Design review of the part built by this model. Coordinates are the model's own, in mm. A direction names the side the tool comes from. Coordinates: 2 decimals unless noted, no trailing zeros. Write each loop counter-clockwise with the first axis right and the second up, starting at its lowest first coordinate (ties: lowest second). Pieces come first, ordered by that corner, then holes.
Q1. Add section B-B, the plane y = 41. Give the boundary of the cut face in (x, z).
Q2. Clearance check with flat-ended pins moving along their axes: pin 1 Ø3 at (y, z) = (10, -4) entering from +X; pin 2 Ø1.8 at (y, z) = (60, -2.5) entering from -X; pin 3 Ø2.5 at (x, z) = (295.5, -3) entering from -Y. State where each tip first meets the part, or that it passes through.
Q3. Add section D-D, the plane z = -1.5. Give the number of separate pieces and of enclosed holes in the cut face, plus the area to 3 significant figures.
Q4. Machinability: for faces 5 (the face through (170, -3, -3)), 6 (the face through (3, 45, -3)), 7 (the face through (294, 57, -3)), 8 (the face through (3, 25, -3)), which of the approach directions +Z, -Z, +X, -X, +Y, -Y give a long, thin tool a straight path to every point of the face, cutting with its end or side? Answer none if there is none.
Q5. Add section A-A, the plane x = 179. Give the boundary of the cut face in (y, z), plus the area to 3 significant figures.
Q6. Add section C-C, the plane x = 80. Give the boundary of the cut face in (y, z), plus the area to 3 significant figures.
Q7. The part is to be moulded in two halves that separate along Y. For faces 1 (the face through (241.102, 46.827, -2.958)), 2 (the face through (68, 0, -3)), 3 (the face through (130, -3, -3)), 4 (the face through (148, 70, -3)), say which applies: +Y half, -Y half, draft (parallel to the pull), parting line (faces both ways), or undercut.
Q8. To check wall thickness, follow probe 1 along Y at (x, z) = (106, -3.85); probe 2 along Y at (x, z) = (131, -4.15); probe 3 along X at (y, z) = (37, -3.7). State the ranges of each line that lie inside material, in increasing order.
from build123d import *

# Parameters (mm, degrees)
SKETCH1_W           = 300
SKETCH1_H           = 70
FRONT_DEPTH         = 6
SKETCH2_W           = 6
SKETCH2_H           = 25
SKETCH2_R           = 4
MOUNT_DEPTH         = 309.116860947
SKETCH3_W           = 40
SKETCH3_H           = 6
BOSS_EXTRUDE1_DEPTH = 6
FILLET_2_R          = 1
SKETCH4_R           = 3
CUT_EXTRUDE1_DEPTH  = 309.116860947
LITE_REACH          = 310.117
SKETCH5_R           = 17.5


with BuildPart() as part:
    # Sketch1 → front (new body)
    with BuildSketch(Plane.XY):
        with Locations((150, 35)):
            Rectangle(SKETCH1_W, SKETCH1_H)
    extrude(amount=-FRONT_DEPTH)

    # Sketch2 → mount (cut, through all)
    with BuildSketch(Plane.XY):
        with Locations((3, 57.5)):
            Rectangle(SKETCH2_W, SKETCH2_H)
        with Locations((3, 12.5)):
            Rectangle(SKETCH2_W, SKETCH2_H)
        with Locations((297, 57.5)):
            Rectangle(SKETCH2_W, SKETCH2_H)
        with Locations((297, 12.5)):
            Rectangle(SKETCH2_W, SKETCH2_H)
        with Locations((80, 60)):
            Circle(SKETCH2_R)
        with Locations((220, 60)):
            Circle(SKETCH2_R)
    extrude(amount=-MOUNT_DEPTH, mode=Mode.SUBTRACT)

    # Sketch3 → Boss-Extrude1 (add)
    with BuildSketch(Plane.XY):
        with Locations((150, -3)):
            Rectangle(SKETCH3_W, SKETCH3_H)
    extrude(amount=-BOSS_EXTRUDE1_DEPTH)

    # fillet 2
    fillet_2_edges = [part.edges().sort_by_distance(p)[0] for p in [
        (0, 45, -3),
        (0, 25, -3),
        (294, 0, -3),
        (300, 25, -3),
        (300, 45, -3),
        (294, 70, -3),
        (6, 0, -3),
        (6, 70, -3),
        (170, -6, -3),
        (130, -6, -3),
    ]]
    fillet(fillet_2_edges, radius=FILLET_2_R)

    # Sketch4 → Cut-Extrude1 (cut, through all)
    with BuildSketch(Plane.XY):
        with Locations((106, 55)):
            Circle(SKETCH4_R)
        with Locations((131, 55)):
            Circle(SKETCH4_R)
        with Locations((106, 30)):
            Circle(SKETCH4_R)
        with Locations((131, 30)):
            Circle(SKETCH4_R)
    extrude(amount=-CUT_EXTRUDE1_DEPTH, mode=Mode.SUBTRACT)

    # Sketch5 → lite (cut, up to next)
    with BuildSketch(Plane.XY, mode=Mode.PRIVATE) as lite_sk1:
        with Locations((46, 35)):
            Circle(SKETCH5_R)
    lite_tool1 = extrude(lite_sk1.sketch, amount=-LITE_REACH, mode=Mode.PRIVATE) & part.part
    # Sketch5 → lite (cut, up to next)
    with BuildSketch(Plane.XY, mode=Mode.PRIVATE) as lite_sk2:
        with Locations((179, 35)):
            Circle(SKETCH5_R)
    lite_tool2 = extrude(lite_sk2.sketch, amount=-LITE_REACH, mode=Mode.PRIVATE) & part.part
    # Sketch5 → lite (cut, up to next)
    with BuildSketch(Plane.XY, mode=Mode.PRIVATE) as lite_sk3:
        with Locations((254, 35)):
            Circle(SKETCH5_R)
    lite_tool3 = extrude(lite_sk3.sketch, amount=-LITE_REACH, mode=Mode.PRIVATE) & part.part
    add(lite_tool1.solids().sort_by_distance((46, 35, 0))[0], mode=Mode.SUBTRACT)
    add(lite_tool2.solids().sort_by_distance((179, 35, 0))[0], mode=Mode.SUBTRACT)
    add(lite_tool3.solids().sort_by_distance((254, 35, 0))[0], mode=Mode.SUBTRACT)


solid = part.part
Here are the results:
1. outline: (0, -6) - (29.56, -6) - (29.56, 0) - (0, 0) - close; (62.44, -6) - (162.56, -6) - (162.56, 0) - (62.44, 0) - close; (195.44, -6) - (237.56, -6) - (237.56, 0) - (195.44, 0) - close; (270.44, -6) - (300, -6) - (300, 0) - (270.44, 0) - close
2. pin 1: stops at x = 294
2. pin 2: stops at x = 6
2. pin 3: stops at y = 25
3. separate pieces: 1
3. enclosed holes: 9
3. area: 17,500 mm2
4. face 5: +Z, -Z, +X, -Y
4. face 6: +Z, -Z, -X, +Y
4. face 7: +Z, -Z, +X, +Y
4. face 8: +Z, -Z, -X, -Y
5. outline: (0, -6) - (17.5, -6) - (17.5, 0) - (0, 0) - close; (52.5, -6) - (70, -6) - (70, 0) - (52.5, 0) - close
5. area: 210 mm2
6. outline: (0, -6) - (56, -6) - (56, 0) - (0, 0) - close; (64, -6) - (70, -6) - (70, 0) - (64, 0) - close
6. area: 372 mm2
7. face 1: undercut
7. face 2: -Y half
7. face 3: draft
7. face 4: +Y half
8. probe 1: y = 0 to 27, 33 to 52, 58 to 70
8. probe 2: y = -6 to 27, 33 to 52, 58 to 70
8. probe 3: x = 0 to 28.61, 63.39 to 161.61, 196.39 to 236.61, 271.39 to 300
